from build123d import *

# Parameters (mm, degrees)
EXTRUDE_1_DEPTH     = 56
SKETCH_2_R          = 7
EXTRUDE_2_DEPTH     = 14
SKETCH_3_R          = 11
EXTRUDE_3_DEPTH     = 8
SKETCH_5_R          = 6
CUT_EXTRUDE_2_DEPTH = 28


with BuildPart() as part:
    # Sketch 1 → Extrude 1 (new body)
    with BuildSketch(Plane.XY):
        Polygon((-13, -7), (-13, 0), (13, 0), (13, -7), (20, -7), (20, 7), (-20, 7), (-20, -7), align=None)
    extrude(amount=EXTRUDE_1_DEPTH)

    # Sketch 2 → Extrude 2 (add)
    with BuildSketch(Plane(origin=(0, 0, 0), x_dir=(-1, 0, 0), z_dir=(0, 0, -1))):
        with BuildLine():
            Line((20, 7), (13.678424719, 35.98340363))
            ThreePointArc((13.678424719, 35.98340363), (0, 47), (-13.678424719, 35.98340363))
            Line((-13.678424719, 35.98340363), (-20, 7))
            Line((-20, 7), (20, 7))
        make_face()
        with Locations((0, 33)):
            Circle(SKETCH_2_R, mode=Mode.SUBTRACT)
    extrude(amount=-EXTRUDE_2_DEPTH)

    # Sketch 3 → Extrude 3 (add)
    with BuildSketch(Plane(origin=(0, 7, 0), x_dir=(1, 0, 0), z_dir=(0, 1, 0))):
        with Locations(Location((0, -36, 0), (0, 0, 270))):
            Circle(SKETCH_3_R)
    extrude(amount=EXTRUDE_3_DEPTH)

    # Sketch 5 → Cut-Extrude 2 (cut)
    with BuildSketch(Plane(origin=(0, 15, 0), x_dir=(1, 0, 0), z_dir=(0, 1, 0))):
        with Locations(Location((0, -35.911740673, 0), (0, 0, 270))):
            Circle(SKETCH_5_R)
    extrude(amount=-CUT_EXTRUDE_2_DEPTH, mode=Mode.SUBTRACT)


solid = part.part
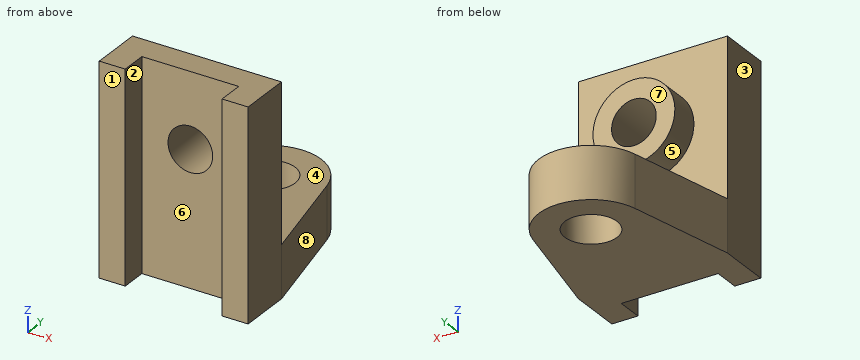
Part model, mm, in its own coordinate system. Face numbers are marked on the shaded views. A direction names the side the tool comes from. Give positions to 0.01 mm unless a question says otherwise; leave off trailing zeros. Order: outer loops, then holes, each group sorted by start corner. A loop starts at its lowest first (then second) coordinate and runs counter-clockwise, first axis right, second up. Notation, with made-up numbers: (-21.5, 76.25) -> (0.5, 76.25) arc R28 ccw to (0.5, 101.25) -> close; hole circle Ø2 at (71, 86.5). An arc over 180 degrees is marked (long way). Use one line per item in the form item = value.
(1) Flat gauge pins, fed straight in: P1, Ø10, axis at x = -4.5, z = 13, coming from the -Y side; P2, Ø24, axis at x = 3.5, z = 36, coming from the +Y side; P3, Ø12, axis at x = -3.5, y = 11, coming from the -Z side; P4, Ø3, axis at x = -15, z = 21, coming from the +Y side. Where does each tip first touch, or does it go through?
Solution:
P1 = 0
P2 = 15
P3 = 0
P4 = 7
(2) Tool access for the marked faces 4, 5, 6, 7 and 8: list every direction of +Z, -Z, +X, -X, +Y, -Y with a clear straight run to the whole face (end or side of a thin tool).
Solution:
face_4 = +X, -X, +Y
face_5 = +Y
face_6 = +Z, -Z, -Y
face_7 = +Z, +X, -X, +Y
face_8 = +Z, -Z, +X, +Y
(3) Pull direction X, two halves, no side cores. Call the marked faces 1, 2 and 3: +X half, -X half, draft (parallel to the pull), parting line (faces both ways), or undercut.
Solution:
face_1 = draft
face_2 = undercut
face_3 = -X half
(4) Saw through at C-C (z = 36). Write the cut outline in (x, y), then the cut area to 3 significant figures.
Solution:
outline = (-20, -7) -> (-13, -7) -> (-13, 0) -> (-6, 0) -> (-6, 15) -> (-11, 15) -> (-11, 7) -> (-20, 7) -> close; (6, 0) -> (13, 0) -> (13, -7) -> (20, -7) -> (20, 7) -> (11, 7) -> (11, 15) -> (6, 15) -> close
area = 374 mm²
(5) Drill centre lines: line 1 (X direction, y = -2.5, z = 11.5); line 2 (Y direction, x = 0, z = 5.75); line 3 (Z direction, x = -3, y = 9). Where is each one in solid material? Low to high. Write a range as from..to.
Solution:
line_1 = -20..-13, 13..20
line_2 = 0..26, 40..47
line_3 = 0..14, 25.42..30.72, 41.11..46.58
(6) Saw through at B-B (y = 5). Write the cut outline in (x, z), then the cut area to 3 significant figures.
Solution:
outline = (-20, 0) -> (20, 0) -> (20, 56) -> (-20, 56) -> close; hole circle Ø12 at (0, 35.91)
area = 2,130 mm²
(7) Saw through at D-D (z = 7). Write the cut outline in (x, y), then the cut area to 3 significant figures.
Solution:
outline = (-20, -7) -> (-13, -7) -> (-13, 0) -> (13, 0) -> (13, -7) -> (20, -7) -> (20, 7) -> (13.68, 35.98) arc R14 ccw to (-13.68, 35.98) -> (-20, 7) -> close; hole circle Ø14 at (0, 33)
area = 1,430 mm²
(8) Saw through at A-A (x = 0). Write the cut outline in (y, z), then the cut area to 3 significant figures.
Solution:
outline = (0, 0) -> (26, 0) -> (26, 14) -> (7, 14) -> (7, 25) -> (15, 25) -> (15, 29.91) -> (0, 29.91) -> close; (0, 41.91) -> (15, 41.91) -> (15, 47) -> (7, 47) -> (7, 56) -> (0, 56) -> close; (40, 0) -> (47, 0) -> (47, 14) -> (40, 14) -> close
area = 752 mm²
